Check sheet for the modelled part. Datum: model origin and axes. Units: mm. Face numbers are marked on the shaded views. A direction names the side the tool comes from. Give positions to 0.01 mm unless a question says otherwise; leave off trailing zeros. Write each loop counter-clockwise with the first axis right and the second up, starting at its lowest first coordinate (ties: lowest second). Pieces come first, ordered by that corner, then holes. Notation, with made-up numbers: (-5.5, 61) -> (11.5, 61) arc R9 ccw to (11.5, 75) -> close; hole circle Ø11 at (40.25, -39.5). An arc over 180 degrees is marked (long way). Return JSON: item names as keys, results as strings.
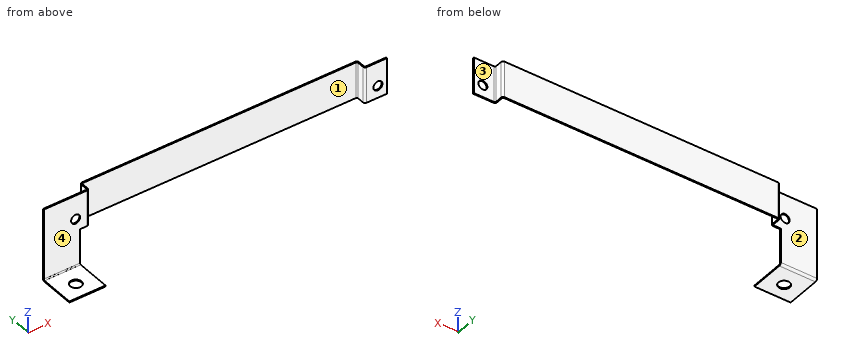
from build123d import *

# Parameters (mm, degrees)
SKETCH1_W                    = 14.25702
SKETCH1_H                    = 25.4
SKETCH1_R                    = 3.175
BASE_FLANGE1_DEPTH           = 0.79375
EDGE_FLANGE1_DEPTH           = 25.4
EDGE_FLANGE2_DEPTH           = 25.4
EDGE_FLANGE3_DEPTH           = 25.4
EDGE_FLANGE4_STRIP_W         = 4.6482
EDGE_FLANGE4_STRIP_H         = 0.79375
EDGE_FLANGE4_STRIP_CUT_DEPTH = 25.4
EDGE_FLANGE4_DEPTH           = 25.4
SKETCH16_R                   = 3.175
CUT_EXTRUDE1_DEPTH           = 236.022644323
SKETCH17_W                   = 25.4
SKETCH17_H                   = 25.7556
TAB1_DEPTH                   = 0.79375
EDGE_FLANGE5_STRIP_W         = 4.6482
EDGE_FLANGE5_STRIP_H         = 0.79375
EDGE_FLANGE5_STRIP_CUT_DEPTH = 25.4
EDGE_FLANGE5_DEPTH           = 25.4
SKETCH25_R                   = 3.96875
CUT_EXTRUDE2_DEPTH           = 242.170466728


# Sheet-metal steps are written as plain solids
with BuildPart() as part:
    # Sketch1 → Base-Flange1 (new body)
    with BuildSketch(Plane(origin=(0, 0, 0), x_dir=(1, 0, 0), z_dir=(0, 1, 0))):
        with Locations((-0.77851, -4.160748346)):
            Rectangle(SKETCH1_W, SKETCH1_H)
        with Locations(Location((0, 0, 0), (0, 0, 270))):
            Circle(SKETCH1_R, mode=Mode.SUBTRACT)
    extrude(amount=-BASE_FLANGE1_DEPTH)

    # Edge-Flange1 section (across the edge) → Edge-Flange1 (add)
    with BuildSketch(Plane(origin=(-8.64362, 0, -8.539251654), x_dir=(1, 0, 0), z_dir=(0, 0, 1))):
        with BuildLine():
            Line((-0.79375, 0.7366), (-0.79375, 5.55625))
            Line((-0.79375, 5.55625), (0, 5.55625))
            Line((0, 5.55625), (0, 0.7366))
            ThreePointArc((0, 0.7366), (0.215745145, 0.215745145), (0.7366, 0))
            Line((0.7366, 0), (0.7366, -0.79375))
            ThreePointArc((0.7366, -0.79375), (-0.345520863, -0.345520863), (-0.79375, 0.7366))
        make_face()
    extrude(amount=EDGE_FLANGE1_DEPTH)

    # Edge-Flange2 section (across the edge) → Edge-Flange2 (add)
    with BuildSketch(Plane(origin=(-9.43737, 6.29285, 16.860748346), x_dir=(0, -1, 0), z_dir=(0, 0, -1))):
        with BuildLine():
            Line((-0.79375, 0.7366), (-0.79375, 192.38595))
            Line((-0.79375, 192.38595), (0, 192.38595))
            Line((0, 192.38595), (0, 0.7366))
            ThreePointArc((0, 0.7366), (0.215745145, 0.215745145), (0.7366, 0))
            Line((0.7366, 0), (0.7366, -0.79375))
            ThreePointArc((0.7366, -0.79375), (-0.345520863, -0.345520863), (-0.79375, 0.7366))
        make_face()
    extrude(amount=EDGE_FLANGE2_DEPTH)

    # Edge-Flange3 section (across the edge) → Edge-Flange3 (add)
    with BuildSketch(Plane(origin=(-202.55992, 6.29285, 16.860748346), x_dir=(1, 0, 0), z_dir=(0, 0, -1))):
        with BuildLine():
            Line((-0.79375, 0.7366), (-0.79375, 7.0866))
            Line((-0.79375, 7.0866), (0, 7.0866))
            Line((0, 7.0866), (0, 0.7366))
            ThreePointArc((0, 0.7366), (0.215745145, 0.215745145), (0.7366, 0))
            Line((0.7366, 0), (0.7366, -0.79375))
            ThreePointArc((0.7366, -0.79375), (-0.345520863, -0.345520863), (-0.79375, 0.7366))
        make_face()
    extrude(amount=EDGE_FLANGE3_DEPTH)

    # Edge-Flange4 strip (across the edge) → Edge-Flange4 strip cut (cut)
    with BuildSketch(Plane(origin=(-203.35367, -0.79375, -8.539251654), x_dir=(0, 1, 0), z_dir=(0, 0, 1))):
        with Locations((-0.79375, -0.396875)):
            Rectangle(EDGE_FLANGE4_STRIP_W, EDGE_FLANGE4_STRIP_H)
    extrude(amount=EDGE_FLANGE4_STRIP_CUT_DEPTH, mode=Mode.SUBTRACT)

    # Edge-Flange4 section (across the edge) → Edge-Flange4 (add)
    with BuildSketch(Plane(origin=(-203.35367, -0.79375, -8.539251654), x_dir=(0, 1, 0), z_dir=(0, 0, 1))):
        with BuildLine():
            Line((0, 0.7366), (0, 30.95625))
            Line((0, 30.95625), (0.79375, 30.95625))
            Line((0.79375, 30.95625), (0.79375, 0.7366))
            ThreePointArc((0.79375, 0.7366), (1.009495145, 0.215745145), (1.53035, 0))
            Line((1.53035, 0), (1.53035, -0.79375))
            ThreePointArc((1.53035, -0.79375), (0.448229137, -0.345520863), (0, 0.7366))
        make_face()
    extrude(amount=EDGE_FLANGE4_DEPTH)

    # Sketch16 → Cut-Extrude1 (cut, through all)
    with BuildSketch(Plane(origin=(0, 0, 0), x_dir=(1, 0, 0), z_dir=(0, 1, 0))):
        with Locations(Location((-211.998031426, 0, 0), (0, 0, 180))):
            Circle(SKETCH16_R)
    extrude(amount=-CUT_EXTRUDE1_DEPTH, mode=Mode.SUBTRACT)

    # Sketch17 → Tab1 (add)
    with BuildSketch(Plane(origin=(0, 0, 0), x_dir=(1, 0, 0), z_dir=(0, 1, 0))):
        with Locations((-221.60992, 21.417051654)):
            Rectangle(SKETCH17_W, SKETCH17_H)
    extrude(amount=-TAB1_DEPTH)

    # Edge-Flange5 strip (across the edge) → Edge-Flange5 strip cut (cut)
    with BuildSketch(Plane(origin=(-234.30992, -0.79375, -34.294851654), x_dir=(0, 0, 1), z_dir=(1, 0, 0))):
        with Locations((-0.79375, -0.396875)):
            Rectangle(EDGE_FLANGE5_STRIP_W, EDGE_FLANGE5_STRIP_H)
    extrude(amount=EDGE_FLANGE5_STRIP_CUT_DEPTH, mode=Mode.SUBTRACT)

    # Edge-Flange5 section (across the edge) → Edge-Flange5 (add)
    with BuildSketch(Plane(origin=(-234.30992, -0.79375, -34.294851654), x_dir=(0, 0, 1), z_dir=(1, 0, 0))):
        with BuildLine():
            Line((0, 0.7366), (0, 24.60625))
            Line((0, 24.60625), (0.79375, 24.60625))
            Line((0.79375, 24.60625), (0.79375, 0.7366))
            ThreePointArc((0.79375, 0.7366), (1.009495145, 0.215745145), (1.53035, 0))
            Line((1.53035, 0), (1.53035, -0.79375))
            ThreePointArc((1.53035, -0.79375), (0.448229137, -0.345520863), (0, 0.7366))
        make_face()
    extrude(amount=EDGE_FLANGE5_DEPTH)

    # Sketch25 → Cut-Extrude2 (cut, through all)
    with BuildSketch(Plane(origin=(0, 0, -34.294851654), x_dir=(-1, 0, 0), z_dir=(0, 0, -1))):
        with Locations(Location((221.60992, -14.23035, 0), (0, 0, 90))):
            Circle(SKETCH25_R)
    extrude(amount=-CUT_EXTRUDE2_DEPTH, mode=Mode.SUBTRACT)


solid = part.part
(1) Set-up check for the marked faces 1, 2, 3 and 4: record each of +Z, -Z, +X, -X, +Y, -Y from which the full face is reachable in a straight line by a thin tool's end or side.
Reply:
{"face 1": "+Z, -Z, -Y", "face 2": "+Z, -Z, -X, +Y", "face 3": "+Z, -Z, +X, +Y", "face 4": "+Z, +X, -X, -Y"}
(2) Thickness scan on L1, parallel to X at y = 2.5, z = -3.5; L2, parallel to Y at x = -119, z = -5; L3, parallel to Y at x = -205.5, z = 6. Record the ranges inside material, lowest first.
Reply:
{"L1": "-203.35 to -202.56, -9.44 to -8.64", "L2": "6.29 to 7.09", "L3": "-0.79 to 0"}
(3) Cross-section at D-D on y = -6. Enter the section's corners in (x, z), then the cut area to 3 significant figures.
Reply:
{"outline": "(-234.31, -34.29) -> (-208.91, -34.29) -> (-208.91, -33.5) -> (-234.31, -33.5) -> close", "area": "20.2 mm^2"}
(4) Depth check by flat-ended pin: pin 1 Ø20.5 at (x, z) = (-60, 7) entering from -Y; pin 2 Ø7 at (x, y) = (-223, -10) entering from +Z; pin 3 Ø1.4 at (y, z) = (4, -1.5) entering from +X; pin 4 Ø4 at (x, z) = (0, 0) entering from -Y. Enter the tip coordinate at first touch or a pass-through.
Reply:
{"pin 1": "y = 6.29", "pin 2": "z = -33.5", "pin 3": "x = -8.64", "pin 4": "through"}
(5) Cross-section at B-B on z = 0. Enter the section's corners in (x, y) (3 decimals), then the cut area to 3 significant figures.
Reply:
{"outline": "(-234.31, -0.794) -> (-215.173, -0.794) -> (-215.173, 0) -> (-234.31, 0) -> close; (-208.823, -0.794) -> (-204.09, -0.794) arc R1.53 ccw to (-202.56, 0.737) -> (-202.56, 5.556) arc R0.737 cw to (-201.823, 6.293) -> (-10.174, 6.293) arc R0.737 cw to (-9.437, 5.556) -> (-9.437, 0.737) arc R1.53 ccw to (-7.907, -0.794) -> (-3.175, -0.794) -> (-3.175, 0) -> (-7.907, 0) arc R0.737 cw to (-8.644, 0.737) -> (-8.644, 5.556) arc R1.53 ccw to (-10.174, 7.087) -> (-201.823, 7.087) arc R1.53 ccw to (-203.354, 5.556) -> (-203.354, 0.737) arc R0.737 cw to (-204.09, 0) -> (-208.823, 0) -> close; (3.175, -0.794) -> (6.35, -0.794) -> (6.35, 0) -> (3.175, 0) -> close", "area": "191 mm^2"}
(6) Cross-section at C-C on x = -153. Enter the section's corners in (y, z).
Reply:
{"outline": "(6.29, -8.54) -> (7.09, -8.54) -> (7.09, 16.86) -> (6.29, 16.86) -> close"}
(7) Cross-section at A-A on x = 0. Enter the section's corners in (y, z) (3 decimals), then the cut area to 3 significant figures.
Reply:
{"outline": "(-0.794, -8.539) -> (0, -8.539) -> (0, -3.175) -> (-0.794, -3.175) -> close; (-0.794, 3.175) -> (0, 3.175) -> (0, 16.861) -> (-0.794, 16.861) -> close", "area": "15.1 mm^2"}
